Solid Edge part; units mm, degrees
sketch "Sketch1" plane through (0, 0, 0) normal (1, 0, 0) x (0, 1, 0)
  circle A0 centre (0, 0) radius 9.43
extrude "Protrusion1" add sketch "Sketch1" along normal blind 1.72
sketch "Sketch2" plane through (1.72, 0, 0) normal (1, 0, 0) x (0, 1, 0)
  circle A0 centre (0, 0) radius 6.22
extrude "Cutout1" cut sketch "Sketch2" against normal through all
chamfer "Chamfer_1" distance 0.5 angle 45 1 edges at (1.72, -9.43, 0)
Here's how the part is built. I have some questions about the finished solid (model axes, mm). Give positions to 0.01 mm unless a question says otherwise; leave off trailing zeros. Loops run counter-clockwise (first coordinate to the right, second up) from the corner with the lowest first, then second, coordinate; pieces in that order, holes last. Notation, with made-up numbers: M 41,-30 L 96,-30 A22 ccw 96,-24 Z; hole C 75.5,-9.5 d4. An arc over 180 degrees is marked long. Return JSON: item names as keys, results as strings.
Item 1: Please list where these lines run through material, in increasing order: line 1 (Z direction, x = 0.6, y = 0); line 2 (Z direction, x = 0.2, y = 4.5); line 3 (Y direction, x = 0.6, z = -1).
A:
{"line 1": "z = -9.43 to -6.22, 6.22 to 9.43", "line 2": "z = -8.29 to -4.29, 4.29 to 8.29", "line 3": "y = -9.38 to -6.14, 6.14 to 9.38"}
Item 2: Imagine slicing it at C-C on x = 0.25. List the corners of the cut face in (y, z) for me, then the cut area to 3 significant figures.
A:
{"outline": "C 0,0 d18.86; hole C 0,0 d12.44", "area": "158 mm^2"}
Item 3: Imagine slicing it at A-A on y = 0. List the corners of the cut face in (x, z) for me.
A:
{"outline": "M 0,-9.43 L 1.22,-9.43 L 1.72,-8.93 L 1.72,-6.22 L 0,-6.22 Z; M 0,6.22 L 1.72,6.22 L 1.72,8.93 L 1.22,9.43 L 0,9.43 Z"}
Item 4: Thinking about a two-plate mould opening in Y: for faces 1 (the cylindrical face through (0.87, -1.35, -6.07)), 2 (the cylindrical face through (0.6, -1.23, -9.35)), 3 (the flat face through (1.72, 1.9, -6.1)), which applies, released by +Y, released by -Y, zero draft, split by the parting line, or undercut?
A:
{"face 1": "undercut", "face 2": "split by the parting line", "face 3": "zero draft"}
